Model file for the job. Use its own axes, mm. Face numbers are marked on the shaded views. A direction names the side the tool comes from. Give positions to 0.01 mm unless a question says otherwise; leave off trailing zeros. Order: outer loops, then holes, each group sorted by start corner. A loop starts at its lowest first (then second) coordinate and runs counter-clockwise, first axis right, second up. Notation, with made-up numbers: M 79,86 L 97,86 A12 cw 97,94 Z; hole C 38,41.25 d9. An arc over 180 degrees is marked long. Return JSON: item names as keys, results as strings. Group by question number.
1. Slice it at A-A on y = 2.25. List the corners of the cut face in (x, z), then the cut area to 3 significant figures.
2. Pin check, flat tips, straight feed: pin 1 (0.9 mm diameter, centred on x = -26.5, y = 3, fed in from -Z); pin 2 (1.5 mm diameter, centred on x = -26.5, y = 2.5, fed in from +Z); pin 3 (0.5 mm diameter, centred on x = -27.5, z = -11, fed in from +Y). Stop position of each tip, or through.
3. Slice it at D-D on y = 4.5. List the corners of the cut face in (x, z) (3 decimals).
4. Two-plate mould, pull along Z, no slides. Class the marked faces 4, 5 and 6: released by +Z, released by -Z, zero draft, split by the parting line, or undercut.
5. Slice it at C-C on z = -12.5. List the corners of the cut face in (x, y), then the cut area to 3 significant figures.
6. Wall check: probe 1 along Z at (x, y) = (-3, 9.75); probe 2 along X at (y, z) = (2.5, -9.75); probe 3 along Y at (x, z) = (-15, -4.5). Give the ranges that are in metal, low to high. Write a range as [from, to].
7. 3-axis set-ups, long thin cutter, end or side, ignore diameter. For the marked faces 1, 2 and 3: which of +Z, -Z, +X, -X, +Y, -Y reach the whole face in a straight line?
8. Slice it at B-B on x = -26. List the corners of the cut face in (y, z).
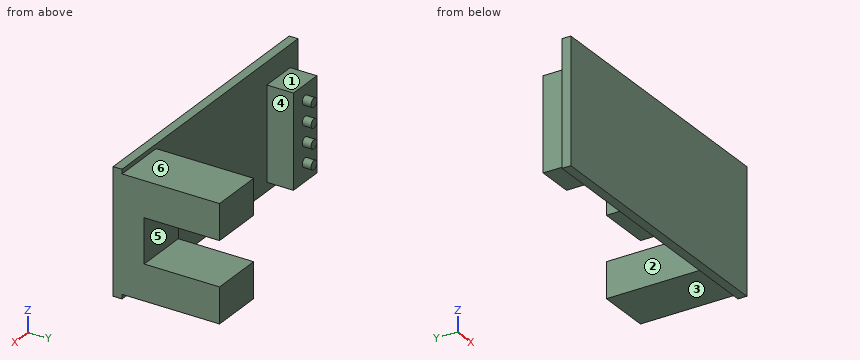
Autodesk Inventor part; units mm, degrees
ref_plane "YZ Plane" through (0, 0, 0) normal (1, 0, 0) x (0, 1, 0)
ref_plane "XZ Plane" through (0, 0, 0) normal (0, 1, 0) x (-1, 0, 0)
ref_plane "XY Plane" through (0, 0, 0) normal (0, 0, 1) x (1, 0, 0)
sketch "草圖1" plane through (0, 0, 0) normal (0, 1, 0) x (-1, 0, 0)
  line L0 (0, 0) -> (31, 0)
  line L1 (31, 0) -> (31, -14)
  line L2 (31, -14) -> (0, -14)
  line L3 (0, -14) -> (0, 0)
  line L4 (6, 0) -> (6, -14)
  line L5 (6, -0.5) -> (0, -0.5)
  line L6 (6, -4.5) -> (0, -4.5)
  line L7 (6, -13.5) -> (0, -13.5)
  line L8 (6, -9.5) -> (0, -9.5)
  line L9 (29.6283, -2.5) -> (25.5101, -2.5)
  line L10 (25.5101, -2.5) -> (25.5101, -13)
  line L11 (25.5101, -13) -> (29.6283, -13)
  line L12 (29.6283, -13) -> (29.6283, -2.5)
  dimension "d0" = 31
  dimension "d1" = 14
  dimension "d2" = 6
  dimension "d3" = 0.5
  dimension "d4" = 4
  dimension "d5" = 4
  dimension "d6" = 0.5
  dimension "d7" = 1
  dimension "d8" = 2.5
extrude "擠出1" add sketch "草圖1" along normal blind 1 contours L0 L4 L5 L3 | L0 L1 L2 L4 | L5 L4 L6 L3 | L6 L4 L8 L3 | L8 L4 L7 L3 | L2 L3 L7 L4 | L12 L11 L10 L9
extrude "擠出2" add sketch "草圖1" along normal blind 12 contours L5 L4 L6 L3 | L8 L4 L7 L3
extrude "擠出3" add sketch "草圖1" along normal blind 4 contours L12 L11 L10 L9
sketch "草圖2" plane through (0, 4, 0) normal (0, 1, 0) x (1, 0, 0)
  circle A0 centre (-27.5692, 4.175) radius 0.5
  line L0 (-29.6283, 2.5) -> (-25.5101, 2.5)
  line L1 (-27.5692, 4.175) -> (-27.5692, 13)
  line L2 (-29.6283, 13) -> (-25.5101, 13)
  circle A1 centre (-27.5692, 6.425) radius 0.5
  circle A2 centre (-27.5692, 8.675) radius 0.5
  circle A3 centre (-27.5692, 10.925) radius 0.5
  point P0 (0, 0)
  point P1 (-27.5692, 2.5)
  dimension "d15" = 1
  dimension "d16" = 1.675
  dimension "d19" = 2.25
extrude "擠出4" add sketch "草圖2" along normal blind 1
extrude "擠出5" add sketch "草圖1" along normal blind 3.5 contours L6 L4 L8 L3
properties part number "LM393" material "MDF Medium Density Fiberboard"
Result:
{
 "1": {"outline": "M -29.63,-13 L -25.51,-13 L -25.51,-2.5 L -29.63,-2.5 Z; M -6,-13.5 L 0,-13.5 L 0,-0.5 L -6,-0.5 Z", "area": "121 mm2"},
 "2": {"pin 1": "stops at z = -13", "pin 2": "stops at z = -2.5", "pin 3": "stops at y = 5"},
 "3": {"outline": "C -27.569,-10.925 d1; C -27.569,-8.675 d1; C -27.569,-6.425 d1; C -27.569,-4.175 d1; M -6,-13.5 L 0,-13.5 L 0,-9.5 L -6,-9.5 Z; M -6,-4.5 L 0,-4.5 L 0,-0.5 L -6,-0.5 Z"},
 "4": {"face 4": "zero draft", "face 5": "undercut", "face 6": "released by +Z"},
 "5": {"outline": "M -31,0 L 0,0 L 0,12 L -6,12 L -6,1 L -25.51,1 L -25.51,4 L -29.63,4 L -29.63,1 L -31,1 Z", "area": "109 mm2"},
 "6": {"probe 1": "z = [-13.5, -9.5], [-4.5, -0.5]", "probe 2": "x = [-29.63, -25.51], [-6, 0]", "probe 3": "y = [0, 1]"},
 "7": {"face 1": "+Z, -X, +Y", "face 2": "+Z, -Z, +Y", "face 3": "-Z, +X, -X, +Y"},
 "8": {"outline": "M 0,-14 L 1,-14 L 1,-13 L 4,-13 L 4,-2.5 L 1,-2.5 L 1,0 L 0,0 Z"}
}
